Answer from the drawing. Dimensions are ordinates in mm from the lowest x, y and z of the part. A direction names the side the tool comes from. Give positions to 0.01 mm unless a question says otherwise; leave off trailing zeros. Write each loop counter-clockwise with the first axis right and the second up, starting at its lowest first coordinate (ties: lowest second). Pieces come first, ordered by that corner, then holes. Notation, with made-up numbers: (5, 80.25) -> (51, 80.25) arc R20 ccw to (51, 86.25) -> close; hole circle Ø9 at (12, 21). An arc over 180 degrees is marked (long way). Put each result on its own line as item: value. Start each with the question number.
1) Find the intervals of material crossed by line 1 along X through (y, z) = (1.1, 6.5) (1 decimal); line 2 along Y through (x, z) = (13.5, 6.5); line 3 along Z through (x, y) = (9.75, 1.5) (1 decimal), in increasing order. Write a range as from..to.
2) For a pull along Y with two mould halves and no side action, classify the marked faces 1, 2 and 3 as released by +Y, released by -Y, zero draft, split by the parting line, or undercut.
3) For the marked faces 4 and 5, determine the directions among +Z, -Z, +X, -X, +Y, -Y from which every point of the face is accessible in a straight line to the end or side of a thin tool.
4) A cutting plane is placed at A-A (y = 6.5). Write down the section's boundary in (x, z) (1 decimal).
5) Flat-ended cylindrical pins translate along their axes: pin 1 Ø1.5 at (y, z) = (5, 9) entering from -X; pin 2 Ø2 at (x, z) = (2, 11) entering from -Y. Find the tip coordinate at first contact, or state that the pin passes through.
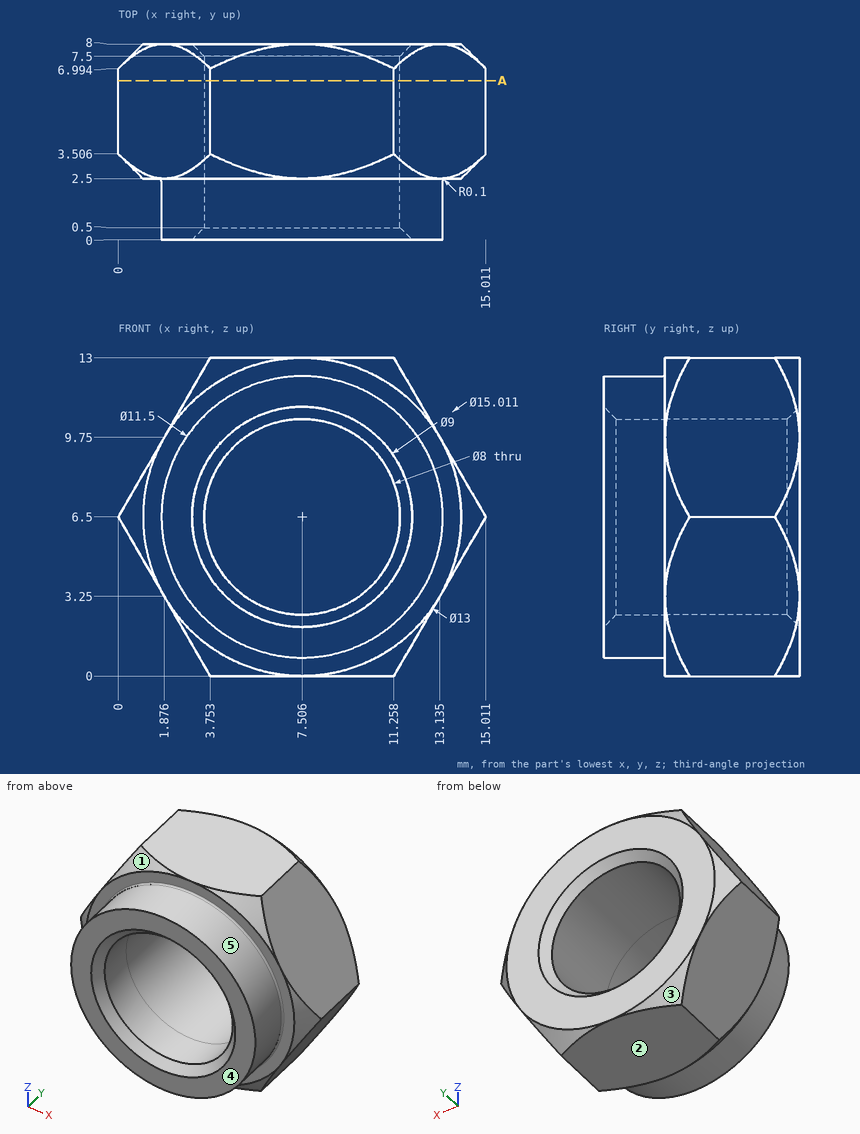
Reply:
1. line 1: x = 1.8..3.5, 11.5..13.3
1. line 2: y = 2.5..8
1. line 3: z = 1.2..3.2, 9.8..11.8
2. face 1: released by -Y
2. face 2: zero draft
2. face 3: released by +Y
3. face 4: +Z, -Z, +X, -X, -Y
3. face 5: -Y
4. outline: (0, 6.5) -> (3.8, 0) -> (11.3, 0) -> (15, 6.5) -> (11.3, 13) -> (3.8, 13) -> close; hole circle Ø8 at (7.5, 6.5)
5. pin 1: stops at x = 1.01
5. pin 2: stops at y = 2.5
